from build123d import *

# Parameters (mm, degrees)
CHANFRO3_SIZE              = 0.2
ESBO_O3_W                  = 12.082799142
ESBO_O3_H                  = 11.091873023
CORTE_EXTRUS_O1_DEPTH      = 1.6
ESBO_O4_W                  = 12.202436568
ESBO_O4_H                  = 8.953230152
CORTE_EXTRUS_O2_DEPTH      = 4
ESBO_O11_R                 = 6.241505963
CORTE_EXTRUS_O5_DEPTH      = 1
ESBO_O5_W                  = 9.712143391
ESBO_O5_H                  = 6.552029914
CORTE_EXTRUS_O3_DEPTH      = 0.5
CORTE_EXTRUS_O4_DEPTH      = 38.504431422
CORTE_EXTRUS_O4_DEPTH_BACK = 38.504431422
CHANFRO6_SIZE              = 1


with BuildPart() as part:
    # Esboço1 → Revolução1 (revolve)
    with BuildSketch(Plane(origin=(0, 0, 0), x_dir=(1, 0, 0), z_dir=(0, 1, 0)), mode=Mode.PRIVATE) as revolu_o1_sk:
        Polygon((35.015459104, 4.5), (35.015459104, 9.5), (28.415459104, 9.5), (28.415459104, 5), (20.75612147, 5), (20.75612147, 4.928604204), (20.515459104, 4.928604204), (20.515459104, 5), (0.015459104, 5), (0.015459104, 3.3), (31.915459104, 3.3), (31.915459104, 5.55), (33.515459104, 5.55), (33.515459104, 4.5), align=None)
    revolve(revolu_o1_sk.sketch.rotate(Axis((0, 0, 0), (1, 0, 0)), 180), axis=Axis((0, 0, 0), (1, 0, 0)))

    # Chanfro3
    # the kernel refuses this chamfer: 0.2 mm, written as the material it takes off along each edge
    with BuildSketch(Plane(origin=(20.75612147, 0, 0), x_dir=(0, 0, 1), z_dir=(0, 1, 0))) as chanfro3_piece_1_section:
        Polygon((5, CHANFRO3_SIZE), (5 - CHANFRO3_SIZE, 0), (5, 0), align=None)
    chanfro3_piece_1 = revolve(axis=Axis((20.75612147, 0, 0), (1, 0, 0)), mode=Mode.PRIVATE)
    chanfro3_piece_1 = chanfro3_piece_1 - Plane(origin=(20.918018136, 0, 0), x_dir=(0, 0, 1), z_dir=(-1, 0, 0)) * Cylinder(4.928604204, 21, mode=Mode.PRIVATE)
    add(chanfro3_piece_1, mode=Mode.SUBTRACT)

    # Esboço3 → Corte-extrusão1 (cut)
    with BuildSketch(Plane(origin=(31.915459104, 0, 0), x_dir=(0, 0, -1), z_dir=(1, 0, 0))):
        with Locations((-6.041399571, 0.003483257)):
            Rectangle(ESBO_O3_W, ESBO_O3_H)
    extrude(amount=CORTE_EXTRUS_O1_DEPTH, mode=Mode.SUBTRACT)

    # Esboço4 → Corte-extrusão2 (cut)
    with BuildSketch(Plane(origin=(31.915459104, 0, 0), x_dir=(0, 0, -1), z_dir=(1, 0, 0))):
        with Locations((-6.101218284, 0.023384924)):
            Rectangle(ESBO_O4_W, ESBO_O4_H)
    extrude(amount=CORTE_EXTRUS_O2_DEPTH, mode=Mode.SUBTRACT)

    # Esboço11 → Corte-extrusão5 (cut)
    with BuildSketch(Plane.ZY.offset(-0.015459104)):
        Circle(ESBO_O11_R)
    extrude(amount=-CORTE_EXTRUS_O5_DEPTH, mode=Mode.SUBTRACT)

    # Esboço5 → Corte-extrusão3 (cut)
    with BuildSketch(Plane(origin=(31.915459104, 0, 0), x_dir=(0, 0, -1), z_dir=(1, 0, 0))):
        with Locations((-4.856071696, 0.023985043)):
            Rectangle(ESBO_O5_W, ESBO_O5_H)
    extrude(amount=-CORTE_EXTRUS_O3_DEPTH, mode=Mode.SUBTRACT)

    # Esboço6 → Corte-extrusão4 (cut, two sides: drawn at the far end of the back side and taken through both)
    with BuildSketch(Plane(origin=(0, 0, 0), x_dir=(1, 0, 0), z_dir=(0, 1, 0)).offset(-CORTE_EXTRUS_O4_DEPTH_BACK)):
        with BuildLine():
            ThreePointArc((29.915459104, -9.5), (32.056996665, -7.305613855), (35.015459104, -6.5))
            add(Edge.make_bspline(
                [(29.915459104, -9.5), (30.631864389, -12.277391552), (37.640288769, -12.30241828), (36.765568572, -6.851347348), (35.015459104, -6.5)],
                knots=[0, 0, 0, 0, 0.632855425, 1, 1, 1, 1], degree=3))
        make_face()
    extrude(amount=CORTE_EXTRUS_O4_DEPTH + CORTE_EXTRUS_O4_DEPTH_BACK, mode=Mode.SUBTRACT)

    # Chanfro6
    chanfro6_edges = [part.edges().sort_by_distance(p)[0] for p in [
        (35.015459104, -4.453230152, 3.573551082),
        (35.015459104, 4.5, 3.25),
        (35.015459104, -0.324395064, -4.488292308),
    ]]
    chamfer(chanfro6_edges, length=CHANFRO6_SIZE)


solid = part.part
CAD build for the part. Positions are in the model's coordinates, mm. A direction names the side the tool comes from. Give positions to 0.01 mm unless a question says otherwise; leave off trailing zeros. Order: outer loops, then holes, each group sorted by start corner. A loop starts at its lowest first (then second) coordinate and runs counter-clockwise, first axis right, second up. Notation, with made-up numbers: (8, 61.5) - (32, 61.5) arc R24 ccw to (32, 74.5) - close; hole circle Ø5 at (64, 77). An arc over 180 degrees is marked (long way). Answer in a Markdown table with one row per item.
1. Saw through at D-D, the plane y = -8. Give the cut face in (x, z), plus the area to 3 significant figures.
Data:
| item | result |
|---|---|
| outline | (28.42, -5.12) - (35.02, -5.12) - (35.02, 5.12) - (28.42, 5.12) - close |
| area | 67.6 mm² |
2. Pull direction Y, two halves, no side cores. Call faces 1 (the cylindrical face through (11, 0, -5)), 2 (the flat face through (1.015, -3.3, -1.2)), 3 (the flat face through (33, -5.542, 4)): pulls with the +Y half, pulls with the -Y half, needs draft (parallel to the pull), parting line crosses it, or undercut.
Data:
| item | result |
|---|---|
| face 1 | parting line crosses it |
| face 2 | needs draft |
| face 3 | undercut |
3. Tool access for faces 4 (the flat face through (33, 5.549, 4)), 5 (the flat face through (34.508, 4.993, 3.339)), 6 (the cylindrical face through (25, 0, -5)), 7 (the cylindrical face through (16.68, -2.23, -2.43)): list every direction of +Z, -Z, +X, -X, +Y, -Y with a clear straight run to the whole face (end or side of a thin tool).
Data:
| item | result |
|---|---|
| face 4 | +Z |
| face 5 | +Z, +X |
| face 6 | -X |
| face 7 | +X, -X |
4. Flat gauge pins, fed straight in: pin 1 (6 mm diameter, centred on x = 28, z = 4.5, fed in from -Y); pin 2 (2 mm diameter, centred on y = 1.5, z = 4, fed in from +X); pin 3 (0.6 mm diameter, centred on x = 34, z = 4, fed in from -Y). Where does each tip first touch, or does it go through?
Data:
| item | result |
|---|---|
| pin 1 | stops at y = -9.38 |
| pin 2 | stops at x = 31.42 |
| pin 3 | stops at y = -8.75 |
5. Saw through at B-B, the plane x = 10. Give the cut face in (y, z).
Data:
| item | result |
|---|---|
| outline | circle Ø10 at (0, 0); hole circle Ø6.6 at (0, 0) |
6. Saw through at C-C, the plane y = 6. Give the cut face in (x, z) (3 decimals).
Data:
| item | result |
|---|---|
| outline | (28.415, -7.365) - (35.015, -7.365) - (35.015, 6.5) arc R5.835 cw to (31.958, 7.365) - (28.415, 7.365) - close |
7. Saw through at A-A, the plane y = 0. Give the cut face in (x, z) (3 decimals), plus the area to 3 significant figures.
Data:
| item | result |
|---|---|
| outline | (1.015, -5) - (20.515, -5) - (20.515, -4.929) - (20.885, -4.929) - (20.956, -5) - (28.415, -5) - (28.415, -9.5) - (35.015, -9.5) - (35.015, -5.5) - (34.015, -4.5) - (33.515, -4.5) - (33.515, -5.55) - (31.915, -5.55) - (31.915, -3.3) - (1.015, -3.3) - close; (1.015, 3.3) - (31.415, 3.3) - (31.415, 7.743) arc R5.835 cw to (29.915, 9.5) - (28.415, 9.5) - (28.415, 5) - (20.956, 5) - (20.885, 4.929) - (20.515, 4.929) - (20.515, 5) - (1.015, 5) - close |
| area | 145 mm² |
8. Probe probe 1 along Y at (x, z) = (21.5, 0); probe 2 along X at (y, z) = (-2, 5); probe 3 along X at (y, z) = (1.25, -3.5). List the from-to ranges inside material, lowest first. Write a range as [from, to].
Data:
| item | result |
|---|---|
| probe 1 | y = [-5, -3.3], [3.3, 5] |
| probe 2 | x = [28.42, 31.42] |
| probe 3 | x = [1.02, 31.92] |
